For this review, take the finished solid that the model builds, in its own axes (mm). Face numbers are marked on the shaded views. Coordinates: 2 decimals unless noted, no trailing zeros. Order: outer loops, then holes, each group sorted by start corner. A loop starts at its lowest first (then second) coordinate and runs counter-clockwise, first axis right, second up. Notation, with made-up numbers: (-26.5, 74) - (32.5, 74) arc R13 cw to (32.5, 80) - close; hole circle Ø10 at (-29.5, 44). An arc over 180 degrees is marked (long way). One line per item, written item: value. Start each with the question number.
(1) Mouldability with a two-part tool opening along Y and no side actions: class the marked faces 1, 2 and 3 as released by +Y, released by -Y, zero draft, split by the parting line, or undercut.
(2) Clearance check with flat-ended pins moving along their axes: pin 1 (1.5 mm diameter, centred on y = 20, z = -6.5, fed in from +X); pin 2 (1 mm diameter, centred on x = -0.5, y = 84.5, fed in from -Z); pin 3 (10 mm diameter, centred on y = 18, z = -6.5, fed in from -X). State where each tip first meets the part, or that it passes through.
(3) Consider section A-A on z = 0. Write out the cut boundary in (x, y).
(4) Consider section B-B on x = -17. Write out the cut boundary in (y, z).
(5) Consider section D-D on x = 29.5. Write out the cut boundary in (y, z), then the cut area to 3 significant figures.
(6) Consider section C-C on y = 51. Write out the cut boundary in (x, z), then the cut area to 3 significant figures.
(7) To check wall thickness, follow line 1 along X through (y, z) = (67, 0); line 2 along Y through (x, z) = (13.5, 0). State the ranges of each line that lie inside material, in increasing order.
```python
from build123d import *

# Parameters (mm, degrees)
SKETCH1_R           = 24.5
SKETCH1_R_2         = 21
SKETCH5_R           = 16
SKETCH5_R_2         = 13.5
BOSS_EXTRUDE3_DEPTH = 58


with BuildPart() as part:
    # Sweep2: sweep along a path in Sketch2
    with BuildLine(Plane.XY) as sweep2_path:
        Line((0, 0), (0, 122))
    # Sketch1 → Sweep2 (sweep)
    with BuildSketch(Plane(origin=(0, 0, 0), x_dir=(1, 0, 0), z_dir=(0, 1, 0))):
        Circle(SKETCH1_R)
        Circle(SKETCH1_R_2, mode=Mode.SUBTRACT)
    sweep(path=sweep2_path.line)

    # Sketch5 → Boss-Extrude3 (add)
    with BuildSketch(Plane(origin=(0, 0, 0), x_dir=(0, 0, -1), z_dir=(1, 0, 0))):
        with Locations(Location((0, 60.289677485, 0), (0, 0, 180))):
            Circle(SKETCH5_R)
        with Locations(Location((0, 60.289677485, 0), (0, 0, 180))):
            Circle(SKETCH5_R_2, mode=Mode.SUBTRACT)
    extrude(amount=BOSS_EXTRUDE3_DEPTH)


solid = part.part
```
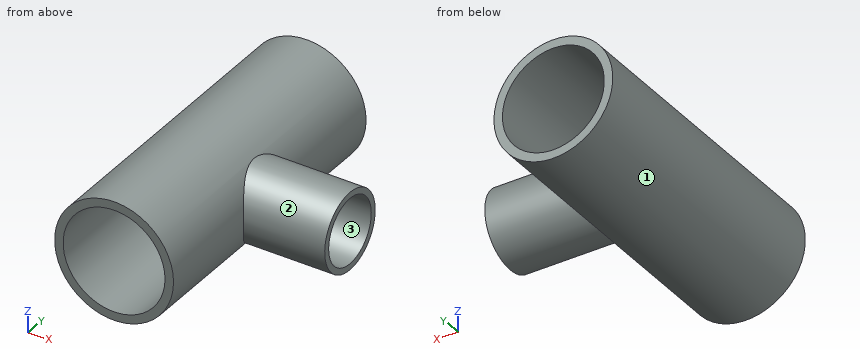
Geometry check:
1. face 1: zero draft
1. face 2: split by the parting line
1. face 3: undercut
2. pin 1: stops at x = 23.82
2. pin 2: stops at z = -24.5
2. pin 3: stops at x = -24.45
3. outline: (-24.5, 0) - (-21, 0) - (-21, 122) - (-24.5, 122) - close; (0, 44.29) - (21, 44.29) - (21, 0) - (24.5, 0) - (24.5, 44.29) - (58, 44.29) - (58, 46.79) - (24.5, 46.79) - (24.5, 73.79) - (58, 73.79) - (58, 76.29) - (24.5, 76.29) - (24.5, 122) - (21, 122) - (21, 76.29) - (0, 76.29) - (0, 73.79) - (21, 73.79) - (21, 46.79) - (0, 46.79) - close
4. outline: (0, -17.64) - (122, -17.64) - (122, -12.33) - (0, -12.33) - close; (0, 12.33) - (122, 12.33) - (122, 17.64) - (0, 17.64) - close
5. outline: circle Ø32 at (60.29, 0); hole circle Ø27 at (60.29, 0)
5. area: 232 mm^2
6. outline: (20.75, -13.03) - (58, -13.03) - (58, -9.8) - (22.46, -9.8) arc R24.5 ccw to (22.46, 9.8) - (58, 9.8) - (58, 13.03) - (20.75, 13.03) arc R24.5 ccw (long way) to start; hole (0, -13.03) - (0, -9.8) - (18.58, -9.8) arc R21 ccw to (18.58, 9.8) - (0, 9.8) - (0, 13.03) - (16.47, 13.03) arc R21 ccw (long way) to (16.47, -13.03) - close
6. area: 849 mm^2
7. line 1: x = -24.5 to -21, 21 to 24.5
7. line 2: y = 44.29 to 46.79, 73.79 to 76.29
